Model file for the job. Use its own axes, mm. Coordinates: 2 decimals unless noted, no trailing zeros. Write each loop counter-clockwise with the first axis right and the second up, starting at its lowest first coordinate (ties: lowest second). Pieces come first, ordered by that corner, then holes. Notation, with made-up numbers: (72, 85) -> (77, 85) arc R8 ccw to (77, 99) -> close; hole circle Ø1 at (24, -6.75). An arc over 180 degrees is marked (long way). Answer as a JSON object with one key per item and string values. Group by question number.
from build123d import *

# Parameters (mm, degrees)
BOSS_EXTRU_1_DEPTH      = 3
BOSS_EXTRU_2_DEPTH      = 1.5
ENL_V_MAT_EXTRU_1_REACH = 266.124
ESQUISSE7_R             = 1.8
CHANFREIN1_SIZE         = 1
CHANFREIN2_SIZE         = 0.25
CONG_1_R                = 0.5
ENL_V_MAT_EXTRU_2_DEPTH = 265.124225417


with BuildPart() as part:
    # Esquisse1 → Boss.-Extru.1 (new body)
    with BuildSketch(Plane.XY):
        with BuildLine():
            Line((-33.076462524, -242.596247682), (-33.076462524, -141.596247682))
            ThreePointArc((-33.076462524, -141.596247682), (-33.955142181, -139.474927339), (-36.076462524, -138.596247682))
            Line((-36.076462524, -138.596247682), (-94.076462524, -138.596247682))
            ThreePointArc((-94.076462524, -138.596247682), (-96.197782868, -139.474927339), (-97.076462524, -141.596247682))
            Line((-97.076462524, -141.596247682), (-97.076462524, -242.596247682))
            ThreePointArc((-97.076462524, -242.596247682), (-96.197782868, -244.717568026), (-94.076462524, -245.596247682))
            Line((-94.076462524, -245.596247682), (-36.076462524, -245.596247682))
            ThreePointArc((-36.076462524, -245.596247682), (-33.955142181, -244.717568026), (-33.076462524, -242.596247682))
        make_face()
    extrude(amount=BOSS_EXTRU_1_DEPTH)

    # Esquisse5 → Boss.-Extru.2 (add)
    with BuildSketch(Plane.XY.offset(3)):
        with BuildLine():
            Line((-40.576462524, -243.096247682), (-40.576462524, -242.596247682))
            ThreePointArc((-40.576462524, -242.596247682), (-39.25844304, -239.414267167), (-36.076462524, -238.096247682))
            Line((-36.076462524, -238.096247682), (-35.576462524, -238.096247682))
            Line((-35.576462524, -238.096247682), (-35.576462524, -146.096247682))
            Line((-35.576462524, -146.096247682), (-36.076462524, -146.096247682))
            ThreePointArc((-36.076462524, -146.096247682), (-39.25844304, -144.778228198), (-40.576462524, -141.596247682))
            Line((-40.576462524, -141.596247682), (-40.576462524, -141.096247682))
            Line((-40.576462524, -141.096247682), (-89.576462524, -141.096247682))
            Line((-89.576462524, -141.096247682), (-89.576462524, -141.596247682))
            ThreePointArc((-89.576462524, -141.596247682), (-90.894482009, -144.778228198), (-94.076462524, -146.096247682))
            Line((-94.076462524, -146.096247682), (-94.576462524, -146.096247682))
            Line((-94.576462524, -146.096247682), (-94.576462524, -238.096247682))
            Line((-94.576462524, -238.096247682), (-94.076462524, -238.096247682))
            ThreePointArc((-94.076462524, -238.096247682), (-90.894482009, -239.414267167), (-89.576462524, -242.596247682))
            Line((-89.576462524, -242.596247682), (-89.576462524, -243.096247682))
            Line((-89.576462524, -243.096247682), (-40.576462524, -243.096247682))
        make_face()
    extrude(amount=BOSS_EXTRU_2_DEPTH)

    # Esquisse7 → Enlèv. mat.-Extru.1 (cut, up to next)
    with BuildSketch(Plane(origin=(0, 0, 0), x_dir=(-1, 0, 0), z_dir=(0, 0, -1)), mode=Mode.PRIVATE) as enl_v_mat_extru_1_sk1:
        with Locations((93.722909134, -242.242694292)):
            Circle(ESQUISSE7_R)
    enl_v_mat_extru_1_tool1 = extrude(enl_v_mat_extru_1_sk1.sketch, amount=-ENL_V_MAT_EXTRU_1_REACH, mode=Mode.PRIVATE) & part.part
    # Esquisse7 → Enlèv. mat.-Extru.1 (cut, up to next)
    with BuildSketch(Plane(origin=(0, 0, 0), x_dir=(-1, 0, 0), z_dir=(0, 0, -1)), mode=Mode.PRIVATE) as enl_v_mat_extru_1_sk2:
        with Locations((93.722909134, -141.949801073)):
            Circle(ESQUISSE7_R)
    enl_v_mat_extru_1_tool2 = extrude(enl_v_mat_extru_1_sk2.sketch, amount=-ENL_V_MAT_EXTRU_1_REACH, mode=Mode.PRIVATE) & part.part
    # Esquisse7 → Enlèv. mat.-Extru.1 (cut, up to next)
    with BuildSketch(Plane(origin=(0, 0, 0), x_dir=(-1, 0, 0), z_dir=(0, 0, -1)), mode=Mode.PRIVATE) as enl_v_mat_extru_1_sk3:
        with Locations((36.430015915, -141.949801073)):
            Circle(ESQUISSE7_R)
    enl_v_mat_extru_1_tool3 = extrude(enl_v_mat_extru_1_sk3.sketch, amount=-ENL_V_MAT_EXTRU_1_REACH, mode=Mode.PRIVATE) & part.part
    # Esquisse7 → Enlèv. mat.-Extru.1 (cut, up to next)
    with BuildSketch(Plane(origin=(0, 0, 0), x_dir=(-1, 0, 0), z_dir=(0, 0, -1)), mode=Mode.PRIVATE) as enl_v_mat_extru_1_sk4:
        with Locations((36.430015915, -242.242694292)):
            Circle(ESQUISSE7_R)
    enl_v_mat_extru_1_tool4 = extrude(enl_v_mat_extru_1_sk4.sketch, amount=-ENL_V_MAT_EXTRU_1_REACH, mode=Mode.PRIVATE) & part.part
    add(enl_v_mat_extru_1_tool1.solids().sort_by_distance((-93.722909, -242.242694, 0))[0], mode=Mode.SUBTRACT)
    add(enl_v_mat_extru_1_tool2.solids().sort_by_distance((-93.722909, -141.949801, 0))[0], mode=Mode.SUBTRACT)
    add(enl_v_mat_extru_1_tool3.solids().sort_by_distance((-36.430016, -141.949801, 0))[0], mode=Mode.SUBTRACT)
    add(enl_v_mat_extru_1_tool4.solids().sort_by_distance((-36.430016, -242.242694, 0))[0], mode=Mode.SUBTRACT)

    # Chanfrein1
    chanfrein1_edges = [part.edges().sort_by_distance(p)[0] for p in [
        (-91.922909134, -242.242694292, 0),
        (-91.922909134, -141.949801073, 0),
        (-34.630015915, -141.949801073, 0),
        (-34.630015915, -242.242694292, 0),
    ]]
    chamfer(chanfrein1_edges, length=CHANFREIN1_SIZE)

    # Chanfrein2
    chanfrein2_edges = [part.edges().sort_by_distance(p)[0] for p in [
        (-65.076462524, -243.096247682, 4.5),
        (-40.576462524, -242.846247682, 4.5),
        (-39.25844304, -239.414267167, 4.5),
        (-35.826462524, -238.096247682, 4.5),
        (-35.576462524, -192.096247682, 4.5),
        (-35.826462524, -146.096247682, 4.5),
        (-39.25844304, -144.778228198, 4.5),
        (-40.576462524, -141.346247682, 4.5),
        (-65.076462524, -141.096247682, 4.5),
        (-89.576462524, -141.346247682, 4.5),
        (-90.894482009, -144.778228198, 4.5),
        (-94.326462524, -146.096247682, 4.5),
        (-94.576462524, -192.096247682, 4.5),
        (-94.326462524, -238.096247682, 4.5),
        (-90.894482009, -239.414267167, 4.5),
        (-89.576462524, -242.846247682, 4.5),
        (-91.922909134, -242.242694292, 3),
        (-91.922909134, -141.949801073, 3),
        (-34.630015915, -141.949801073, 3),
        (-34.630015915, -242.242694292, 3),
    ]]
    chamfer(chanfrein2_edges, length=CHANFREIN2_SIZE)

    # Congé1
    cong_1_edges = [part.edges().sort_by_distance(p)[0] for p in [
        (-94.576462524, -238.096247682, 3.625),
        (-89.576462524, -243.096247682, 3.625),
        (-35.576462524, -146.096247682, 3.625),
        (-40.576462524, -141.096247682, 3.625),
        (-89.576462524, -141.096247682, 3.625),
        (-94.576462524, -146.096247682, 3.625),
        (-35.576462524, -238.096247682, 3.625),
        (-40.576462524, -243.096247682, 3.625),
    ]]
    fillet(cong_1_edges, radius=CONG_1_R - 0.0001)  # a hair under: the kernel refuses the full size

    # Esquisse8 → Enlèv. mat.-Extru.2 (cut, through all)
    with BuildSketch(Plane.XY.offset(4.5)):
        with BuildLine():
            Line((-68.076462524, -171.971247682), (-68.076462524, -168.971247682))
            ThreePointArc((-68.076462524, -168.971247682), (-65.076462524, -157.77509526), (-62.076462524, -168.971247682))
            Line((-62.076462524, -168.971247682), (-62.076462524, -171.971247682))
            ThreePointArc((-62.076462524, -171.971247682), (-65.076462524, -174.971247682), (-68.076462524, -171.971247682))
        make_face()
        with BuildLine():
            Line((-68.076462524, -217.971247682), (-68.076462524, -214.971247682))
            ThreePointArc((-68.076462524, -214.971247682), (-65.076462524, -203.77509526), (-62.076462524, -214.971247682))
            Line((-62.076462524, -214.971247682), (-62.076462524, -217.971247682))
            ThreePointArc((-62.076462524, -217.971247682), (-65.076462524, -220.971247682), (-68.076462524, -217.971247682))
        make_face()
    extrude(amount=-ENL_V_MAT_EXTRU_2_DEPTH, mode=Mode.SUBTRACT)


solid = part.part
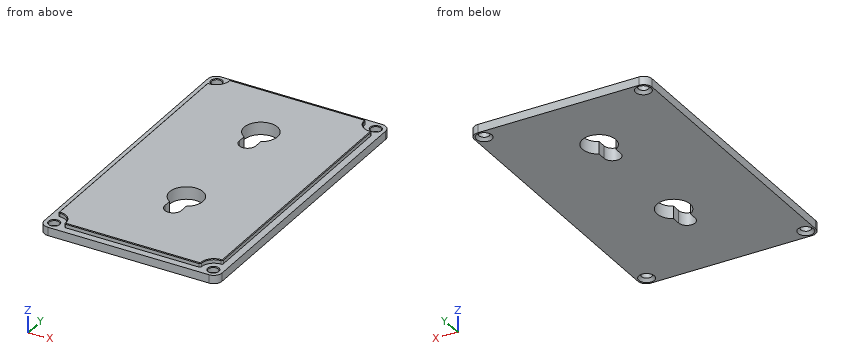
(1) Cut at C-C on z = 1.75. List the corners of the cut face in (x, y), plus the area to 3 significant figures.
(2) Wall check: probe 1 along Y at (x, z) = (-61, 2.25); probe 2 along X at (y, z) = (-171, 3.2); probe 3 along X at (y, z) = (-241, 1.45). Give the ranges that are in metal, low to high.
(3) Cut at B-B on x = -66.5. List the corners of the cut face in (y, z).
(4) Cut at D-D on x = -76. List the corners of the cut face in (y, z).
(5) Cut at A-A on y = -229. List the corners of the cut face in (x, z).
(6) Pin check, flat tip, straight feed: pin 1 (4 mm diameter, centred on x = -36.43, y = -242.24, fed in from -Z). Stop position of the tip, or through.
Results found:
{
 "1": {"outline": "(-97.08, -242.6) arc R3 ccw to (-94.08, -245.6) -> (-36.08, -245.6) arc R3 ccw to (-33.08, -242.6) -> (-33.08, -141.6) arc R3 ccw to (-36.08, -138.6) -> (-94.08, -138.6) arc R3 ccw to (-97.08, -141.6) -> close; hole circle Ø3.6 at (-93.72, -242.24); hole circle Ø3.6 at (-93.72, -141.95); hole (-68.08, -217.97) arc R3 ccw to (-62.08, -217.97) -> (-62.08, -214.97) arc R6 ccw (long way) to (-68.08, -214.97) -> close; hole (-68.08, -171.97) arc R3 ccw to (-62.08, -171.97) -> (-62.08, -168.97) arc R6 ccw (long way) to (-68.08, -168.97) -> close; hole circle Ø3.6 at (-36.43, -242.24); hole circle Ø3.6 at (-36.43, -141.95)", "area": "6,520 mm²"},
 "2": {"probe 1": "y = -245.6 to -214.18, -205.37 to -168.18, -159.37 to -138.6", "probe 2": "x = -94.58 to -68.08, -62.08 to -35.58", "probe 3": "x = -97.08 to -95.03, -92.42 to -37.73, -35.13 to -33.08"},
 "3": {"outline": "(-245.6, 0) -> (-220.61, 0) -> (-220.61, 4.5) -> (-242.85, 4.5) -> (-243.1, 4.25) -> (-243.1, 3) -> (-245.6, 3) -> close; (-203.95, 0) -> (-174.61, 0) -> (-174.61, 4.5) -> (-203.95, 4.5) -> close; (-157.95, 0) -> (-138.6, 0) -> (-138.6, 3) -> (-141.1, 3) -> (-141.1, 4.25) -> (-141.35, 4.5) -> (-157.95, 4.5) -> close"},
 "4": {"outline": "(-245.6, 0) -> (-138.6, 0) -> (-138.6, 3) -> (-141.1, 3) -> (-141.1, 4.25) -> (-141.35, 4.5) -> (-242.85, 4.5) -> (-243.1, 4.25) -> (-243.1, 3) -> (-245.6, 3) -> close"},
 "5": {"outline": "(-97.08, 0) -> (-33.08, 0) -> (-33.08, 3) -> (-35.58, 3) -> (-35.58, 4.25) -> (-35.83, 4.5) -> (-94.33, 4.5) -> (-94.58, 4.25) -> (-94.58, 3) -> (-97.08, 3) -> close"},
 "6": {"pin 1": "stops at z = 0.8"}
}
